The listing builds one solid part. Answer for the finished solid, in the listing's coordinates (mm). Coordinates: 2 decimals unless noted, no trailing zeros. Write each loop counter-clockwise with the first axis right and the second up, starting at its lowest first coordinate (ties: lowest second). Pieces come first, ordered by that corner, then holes. Notation, with made-up numbers: M 67.5,6 L 85.5,6 A31 ccw 85.5,43 Z; hole C 31.5,77.5 d1. An arc over 180 degrees is marked long. Put each result on its own line as item: value. Start each with the question number.
```python
from build123d import *

# Parameters (mm, degrees)
ESQUISSE1_R      = 35
EXTRUSION1_DEPTH = 30
CHANFREIN1_SIZE  = 2
CHANFREIN2_SIZE  = 2


with BuildPart() as part:
    # Esquisse1 → Extrusion1 (new body)
    with BuildSketch(Plane.XY):
        Circle(ESQUISSE1_R)
    extrude(amount=EXTRUSION1_DEPTH)

    # Chanfrein1
    chanfrein1_edges = [part.edges().sort_by_distance(p)[0] for p in [
        (-35, 0, 30),
    ]]
    chamfer(chanfrein1_edges, length=CHANFREIN1_SIZE)

    # Chanfrein2
    chanfrein2_edges = [part.edges().sort_by_distance(p)[0] for p in [
        (-35, 0, 0),
    ]]
    chamfer(chanfrein2_edges, length=CHANFREIN2_SIZE)


solid = part.part
```
1) Straight lines are drawn through the part: probe 1 along Y at (x, z) = (0.5, 14.5); probe 2 along Y at (x, z) = (12.5, 19); probe 3 along X at (y, z) = (18, 9.25). For each, find the intervals that lie inside material, in ascending order.
2) A cutting plane is placed at A-A on z = 24.25. Write down the section's boundary in (x, y).
3) Given pin 1 Ø6 at (x, z) = (23, 22.5) entering from +Y; pin 2 Ø2 at (x, y) = (-23.5, -13) entering from -Z; pin 3 Ø3 at (x, z) = (-10.5, 21) entering from -Y; pin 4 Ø6 at (x, z) = (5, 11.5) entering from -Y, each flat-ended and moving along its own axis, determine where each tip first touches the part or whether it passes through.
Answers follow:
1. probe 1: y = -35 to 35
1. probe 2: y = -32.69 to 32.69
1. probe 3: x = -30.02 to 30.02
2. outline: C 0,0 d70
3. pin 1: stops at y = 28.72
3. pin 2: stops at z = 0
3. pin 3: stops at y = -33.82
3. pin 4: stops at y = -34.94
